Here's how the part is built. I have some questions about the finished solid (model axes, mm). A direction names the side the tool comes from. Round coordinates to 2 decimals unless told otherwise and drop trailing zeros. Loops run counter-clockwise (first coordinate to the right, second up) from the corner with the lowest first, then second, coordinate; pieces in that order, holes last. Notation, with made-up numbers: M 89,33 L 115,33 A26 ccw 115,49 Z; hole C 30.5,79.25 d10. An arc over 180 degrees is marked long. Answer as a JSON object with one key per item and string values.
from build123d import *

# Parameters (mm, degrees)
F0_W         = 25
F0_H         = 12
F0_R         = 2
F1_DEPTH     = 5
F2_R         = 2
F3_R         = 2
F4_R         = 2
F5_R         = 2
F6_T1_DEPTH  = 1
F6_T6_DEPTH  = 2
F6_T12_DEPTH = 2
F6_S17_W     = 2
F6_S17_H     = 2
F6_T18_DEPTH = 2
F6_S23_W     = 2
F6_S23_H     = 2
F6_T24_DEPTH = 2
F7_T1_DEPTH  = 1
F7_S5_W      = 2
F7_S5_H      = 2
F7_T6_DEPTH  = 2
F7_S11_W     = 2
F7_S11_H     = 2
F7_T12_DEPTH = 2
F8_R         = 2


# Not quite as in the source:
# - a fillet or chamfer that OpenCascade refuses, or shapes differently, is made with other operations: its cross-section is extruded or revolved along the edge and cut away or added


with BuildPart() as f1:
    # F0 (on Top) → F1 (new body)
    with BuildSketch(Plane.XY):
        with Locations((-12.5, 6)):
            Rectangle(F0_W, F0_H)
        with Locations((-19, 6)):
            Circle(F0_R, mode=Mode.SUBTRACT)
        with Locations((-11, 6)):
            Circle(F0_R, mode=Mode.SUBTRACT)
        with Locations((-3, 6)):
            Circle(F0_R, mode=Mode.SUBTRACT)
        Polygon((0, 12), (0, 0), (42.2861679354, -15.3909064497), (57.2861679354, -15.3909064497), (57.2861679354, -3.3909064497), (42.2861679354, -3.3909064497), align=None)
        with Locations((44.1906489432, -9.3909064497)):
            Circle(F0_R, mode=Mode.SUBTRACT)
        with Locations((52.0649450129, -9.3909064497)):
            Circle(F0_R, mode=Mode.SUBTRACT)
    extrude(amount=F1_DEPTH)

    # F2
    f2_edges = [f1.edges().sort_by_distance(p)[0] for p in [
        (-12.5, 0, 0),
        (-25, 6, 0),
        (-12.5, 12, 0),
        (21.143084, 4.304547, 0),
        (49.786168, -3.390906, 0),
        (57.286168, -9.390906, 0),
        (49.786168, -15.390906, 0),
        (21.143084, -7.695453, 0),
    ]]
    fillet(f2_edges, radius=F2_R)

    # F3
    f3_edges = [f1.edges().sort_by_distance(p)[0] for p in [
        (57.286168, -9.390906, 5),
        (49.786168, -15.390906, 5),
        (21.143084, -7.695453, 5),
        (-12.5, 0, 5),
        (-25, 6, 5),
        (-12.5, 12, 5),
        (21.143084, 4.304547, 5),
        (49.786168, -3.390906, 5),
    ]]
    fillet(f3_edges, radius=F3_R)

    # F4
    f4_edges = [f1.edges().sort_by_distance(p)[0] for p in [
        (42.181922, -3.982115, 4.419615),
        (42.286168, -3.390906, 2.5),
        (42.181922, -3.982115, 0.580385),
    ]]
    fillet(f4_edges, radius=F4_R)

    # F5
    f5_edges = [f1.edges().sort_by_distance(p)[0] for p in [
        (0.104246, 0.591209, 4.419615),
        (0, 0, 2.5),
        (0.104246, 0.591209, 0.580385),
    ]]
    fillet(f5_edges, radius=F5_R)

    # F6: fillet of radius 2 on 6 edges, made by hand

    # F6_s2 → F6_t1 (cut)
    with BuildSketch(Plane.XY.offset(2)):
        with BuildLine():
            ThreePointArc((41.9547816101, -15.2702916912), (42.2915255414, -15.3605219557), (42.6388218968, -15.3909064497))
            Line((42.6388218968, -15.3909064497), (42.2861679354, -15.3909064497))
            Line((42.2861679354, -15.3909064497), (41.9547816101, -15.2702916912))
        make_face()
        with BuildLine():
            ThreePointArc((55.2861679354, -15.3909064497), (56.7003814977, -14.805120012), (57.2861679354, -13.3909064497))
            Line((57.2861679354, -13.3909064497), (57.2861679354, -15.3909064497))
            Line((57.2861679354, -15.3909064497), (55.2861679354, -15.3909064497))
        make_face()
    extrude(amount=F6_T1_DEPTH, mode=Mode.SUBTRACT)


with BuildPart() as f6_tool4:
    # F6_s5 → F6_t6 (new body)
    with BuildSketch(Plane.XY.offset(3)):
        Polygon((42.6388218968, -13.3909064497), (41.9547816101, -15.2702916912), (42.2861679354, -15.3909064497), (42.6388218968, -15.3909064497), align=None)
    extrude(amount=F6_T6_DEPTH)

    # F6_s7 → F6_t8 (revolve, cut)
    with BuildSketch(Plane(origin=(42.6388218968, -13.3909064497, 3), x_dir=(0.1736481777, 0.984807753, 0), z_dir=(0.984807753, -0.1736481777, 0))):
        with BuildLine():
            ThreePointArc((0, -2), (2, 0), (0, 2))
            Line((0, 2), (0, -2))
        make_face()
    revolve(axis=Axis((42.6388218968, -13.3909064497, 3), (0, 0, 1)), mode=Mode.SUBTRACT)


with BuildPart() as f1_1:
    add(f1.part)

    # F6_t3: cut F6_tool4
    add(f6_tool4.part, mode=Mode.SUBTRACT)


with BuildPart() as f6_tool10:
    # F6_s11 → F6_t12 (new body)
    with BuildSketch(Plane.XY.offset(2)):
        Polygon((42.6388218968, -13.3909064497), (41.9547816101, -15.2702916912), (42.2861679354, -15.3909064497), (42.6388218968, -15.3909064497), align=None)
    extrude(amount=-F6_T12_DEPTH)

    # F6_s13 → F6_t14 (revolve, cut)
    with BuildSketch(Plane(origin=(42.6388218968, -13.3909064497, 2), x_dir=(0.1736481777, 0.984807753, 0), z_dir=(-0.984807753, 0.1736481777, 0))):
        with BuildLine():
            ThreePointArc((0, -2), (2, 0), (0, 2))
            Line((0, 2), (0, -2))
        make_face()
    revolve(axis=Axis((42.6388218968, -13.3909064497, 2), (0, 0, -1)), mode=Mode.SUBTRACT)


with BuildPart() as f1_2:
    add(f1_1.part)

    # F6_t9: cut F6_tool10
    add(f6_tool10.part, mode=Mode.SUBTRACT)


with BuildPart() as f6_tool16:
    # F6_s17 → F6_t18 (new body)
    with BuildSketch(Plane.XZ.offset(13.3909064497)):
        with Locations((56.2861679354, 4)):
            Rectangle(F6_S17_W, F6_S17_H)
    extrude(amount=F6_T18_DEPTH)

    # F6_s19 → F6_t20 (revolve, cut)
    with BuildSketch(Plane(origin=(55.2861679354, -13.3909064497, 3), x_dir=(-0.7071067812, 0, -0.7071067812), z_dir=(-0.7071067812, 0, 0.7071067812))):
        with BuildLine():
            ThreePointArc((0, -2), (2, 0), (0, 2))
            Line((0, 2), (0, -2))
        make_face()
    revolve(axis=Axis((55.2861679354, -13.3909064497, 3), (0, -1, 0)), mode=Mode.SUBTRACT)


with BuildPart() as f1_3:
    add(f1_2.part)

    # F6_t15: cut F6_tool16
    add(f6_tool16.part, mode=Mode.SUBTRACT)


with BuildPart() as f6_tool22:
    # F6_s23 → F6_t24 (new body)
    with BuildSketch(Plane.XZ.offset(13.3909064497)):
        with Locations((56.2861679354, 1)):
            Rectangle(F6_S23_W, F6_S23_H)
    extrude(amount=F6_T24_DEPTH)

    # F6_s25 → F6_t26 (revolve, cut)
    with BuildSketch(Plane(origin=(55.2861679354, -13.3909064497, 2), x_dir=(-0.7071067812, 0, 0.7071067812), z_dir=(0.7071067812, 0, 0.7071067812))):
        with BuildLine():
            ThreePointArc((0, -2), (2, 0), (0, 2))
            Line((0, 2), (0, -2))
        make_face()
    revolve(axis=Axis((55.2861679354, -13.3909064497, 2), (0, -1, 0)), mode=Mode.SUBTRACT)


with BuildPart() as f1_4:
    add(f1_3.part)

    # F6_t21: cut F6_tool22
    add(f6_tool22.part, mode=Mode.SUBTRACT)

    # F7: fillet of radius 2 on 3 edges, made by hand

    # F7_s2 → F7_t1 (cut)
    with BuildSketch(Plane.XY.offset(2)):
        with BuildLine():
            ThreePointArc((57.2861679354, -5.3909064497), (56.7003814977, -3.9766928873), (55.2861679354, -3.3909064497))
            Line((55.2861679354, -3.3909064497), (57.2861679354, -3.3909064497))
            Line((57.2861679354, -3.3909064497), (57.2861679354, -5.3909064497))
        make_face()
    extrude(amount=F7_T1_DEPTH, mode=Mode.SUBTRACT)


with BuildPart() as f7_tool4:
    # F7_s5 → F7_t6 (new body)
    with BuildSketch(Plane.YZ.offset(55.2861679354)):
        with Locations((-4.3909064497, 4)):
            Rectangle(F7_S5_W, F7_S5_H)
    extrude(amount=F7_T6_DEPTH)

    # F7_s7 → F7_t8 (revolve, cut)
    with BuildSketch(Plane(origin=(55.2861679354, -5.3909064497, 3), x_dir=(0, -0.7071067812, -0.7071067812), z_dir=(0, -0.7071067812, 0.7071067812))):
        with BuildLine():
            ThreePointArc((0, -2), (2, 0), (0, 2))
            Line((0, 2), (0, -2))
        make_face()
    revolve(axis=Axis((55.2861679354, -5.3909064497, 3), (1, 0, 0)), mode=Mode.SUBTRACT)


with BuildPart() as f1_5:
    add(f1_4.part)

    # F7_t3: cut F7_tool4
    add(f7_tool4.part, mode=Mode.SUBTRACT)


with BuildPart() as f7_tool10:
    # F7_s11 → F7_t12 (new body)
    with BuildSketch(Plane.YZ.offset(55.2861679354)):
        with Locations((-4.3909064497, 1)):
            Rectangle(F7_S11_W, F7_S11_H)
    extrude(amount=F7_T12_DEPTH)

    # F7_s13 → F7_t14 (revolve, cut)
    with BuildSketch(Plane(origin=(55.2861679354, -5.3909064497, 2), x_dir=(0, -0.7071067812, 0.7071067812), z_dir=(0, 0.7071067812, 0.7071067812))):
        with BuildLine():
            ThreePointArc((0, -2), (2, 0), (0, 2))
            Line((0, 2), (0, -2))
        make_face()
    revolve(axis=Axis((55.2861679354, -5.3909064497, 2), (1, 0, 0)), mode=Mode.SUBTRACT)


with BuildPart() as f1_6:
    add(f1_5.part)

    # F7_t9: cut F7_tool10
    add(f7_tool10.part, mode=Mode.SUBTRACT)

    # F8
    f8_edges = [f1_6.edges().sort_by_distance(p)[0] for p in [
        (-0.104246, 11.408791, 0.580385),
        (-0.104246, 11.408791, 4.419615),
        (0, 12, 2.5),
    ]]
    fillet(f8_edges, radius=F8_R)


solid = f1_6.part
Item 1: If we mould it in two halves opening along Y, with no side actions, what happens to faces 1 (the face through (20.983, 3.756, 0.601)), 2 (the face through (-3, 8, 2)), 3 (the face through (56.716, -9.335, 0.601))? For each: pulls with the +Y half, pulls with the -Y half, needs draft (parallel to the pull), parting line crosses it, or undercut.
Resolved:
{"face 1": "pulls with the +Y half", "face 2": "undercut", "face 3": "needs draft"}
Item 2: I want a section at C-C, the plane x = -2.5. Please give me the cut outline in (y, z), then the cut area to 3 significant figures.
Resolved:
{"outline": "M 0,2 A2 ccw 2,0 L 4.06,0 L 4.06,5 L 2,5 A2 ccw 0,3 Z; M 7.94,0 L 10,0 A2 ccw 12,2 L 12,3 A2 ccw 10,5 L 7.94,5 Z", "area": "37.2 mm²"}
Item 3: On a 3-axis mill with a long thin cutter (end or side, diameter ignored), from which of +Z, -Z, +X, -X, +Y, -Y can I reach the whole of each face in a straight line? I mean faces 4 (the face through (-12.15, 0.57, 0.6)), 5 (the face through (-24.43, 6.08, 4.4)), 6 (the face through (21.43, 4.2, 2.49)), 7 (the face through (48.52, -3.96, 0.6)), 8 (the face through (-12.15, 0.57, 4.4)). Say none if no direction works.
Resolved:
{"face 4": "-Z, -X, -Y", "face 5": "+Z, -X, +Y, -Y", "face 6": "+Z, -Z, +X, +Y", "face 7": "-Z, +X, +Y", "face 8": "+Z, -X, -Y"}
Item 4: I want a section at B-B, the plane z = 3.85. State how many separate pieces and enclosed holes the cut face has, then the cut area to 3 significant figures.
Resolved:
{"separate pieces": "1", "enclosed holes": "5", "area": "887 mm²"}
Item 5: I want a section at A-A, the plane x = -19. Please give me the cut outline in (y, z), then the cut area to 3 significant figures.
Resolved:
{"outline": "M 0,2 A2 ccw 2,0 L 4,0 L 4,5 L 2,5 A2 ccw 0,3 Z; M 8,0 L 10,0 A2 ccw 12,2 L 12,3 A2 ccw 10,5 L 8,5 Z", "area": "36.6 mm²"}
Item 6: Please list where these lines run through material, in increasing order: probe 1 along Y at (x, z) = (-3, 3.15); probe 2 along Y at (x, z) = (45, 4.55); probe 3 along Y at (x, z) = (13.5, 4.1). Write a range as from..to.
Resolved:
{"probe 1": "0.01..4, 8..11.99", "probe 2": "-14.65..-11.22, -7.56..-4.13", "probe 3": "-4.56..6.74"}
Item 7: I'm going to push flat-ended pins straight in: pin 1 Ø12 at (x, y) = (38.5, 2.5) entering from +Z; pin 2 Ø0.8 at (x, z) = (48, 2.5) entering from +Y; pin 3 Ø0.8 at (x, z) = (-8.5, 2.5) entering from -Y. Where does each tip first touch, or does it pass through?
Resolved:
{"pin 1": "z = 4.99", "pin 2": "y = -3.39", "pin 3": "y = 0"}
